```python
from build123d import *

# Parameters (mm, degrees)
SKETCH_1_R      = 1.5
EXTRUDE_1_DEPTH = 42
SKETCH_2_R      = 1.25
EXTRUDE_2_DEPTH = 0.8
SKETCH_3_R      = 1.5
EXTRUDE_3_DEPTH = 3
SKETCH_4_R      = 2.8
EXTRUDE_4_DEPTH = 1.3
FILLET_1_R      = 1


with BuildPart() as part:
    # 草图1 → 凸台-拉伸1 (new body)
    with BuildSketch(Plane(origin=(0, 0, 0), x_dir=(1, 0, 0), z_dir=(0, 1, 0))):
        with Locations(Location((0, 0, 0), (0, 0, 90))):
            Circle(SKETCH_1_R)
    extrude(amount=EXTRUDE_1_DEPTH)

    # 草图2 → 凸台-拉伸2 (add)
    with BuildSketch(Plane(origin=(0, 42, 0), x_dir=(1, 0, 0), z_dir=(0, 1, 0))):
        with Locations(Location((0, 0, 0), (0, 0, 270))):
            Circle(SKETCH_2_R)
    extrude(amount=EXTRUDE_2_DEPTH)

    # 草图3 → 凸台-拉伸3 (add)
    with BuildSketch(Plane(origin=(0, 42.8, 0), x_dir=(1, 0, 0), z_dir=(0, 1, 0))):
        with Locations(Location((0, 0, 0), (0, 0, 90))):
            Circle(SKETCH_3_R)
    extrude(amount=EXTRUDE_3_DEPTH)

    # 草图4 → 凸台-拉伸4 (add)
    with BuildSketch(Plane.XZ):
        with Locations(Location((0, 0, 0), (0, 0, 270))):
            Circle(SKETCH_4_R)
    extrude(amount=EXTRUDE_4_DEPTH)

    # 圆角1
    fillet_1_edges = [part.edges().sort_by_distance(p)[0] for p in [
        (0, -1.3, 2.8),
    ]]
    fillet(fillet_1_edges, radius=FILLET_1_R)


solid = part.part
```
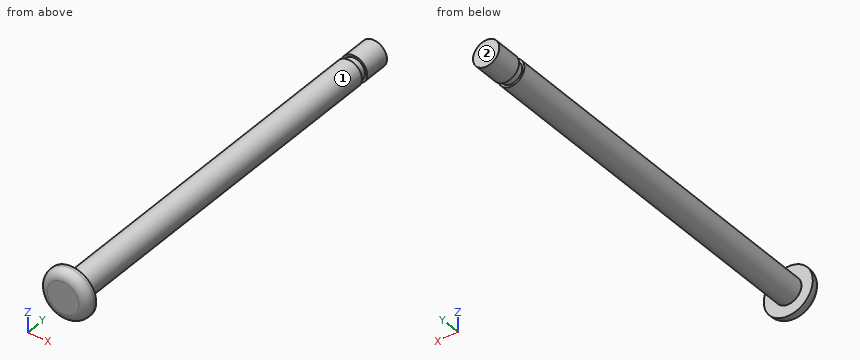
Model file for the job. Use its own axes, mm. Face numbers are marked on the shaded views. A direction names the side the tool comes from. Round coordinates to 2 decimals unless told otherwise and drop trailing zeros. Order: outer loops, then holes, each group sorted by start corner. A loop starts at its lowest first (then second) coordinate and runs counter-clockwise, first axis right, second up. Notation, with made-up numbers: M 72,62 L 77,62 A25 cw 77,92 Z; hole C 23.5,0 d6. An arc over 180 degrees is marked long. Use CSV: the item, a comma, the result in double quotes.
Item 1: Which spindle directions (+Z, -Z, +X, -X, +Y, -Y) get a long thin tool onto all of the face, cutting with end or side? Do the marked faces 1 and 2. Say none if no direction does.
Worked answers:
face 1,"+Y"
face 2,"+Z, -Z, +X, -X, +Y"
Item 2: Saw through at C-C (y = 13.5). List the corners of the cut face in (x, z), plus the area to 3 significant figures.
Worked answers:
outline,"C 0,0 d3"
area,"7.07 mm²"
Item 3: Saw through at B-B (z = 0). List the corners of the cut face in (x, y).
Worked answers:
outline,"M -2.8,-0.3 A1 ccw -1.8,-1.3 L 1.8,-1.3 A1 ccw 2.8,-0.3 L 2.8,0 L 1.5,0 L 1.5,42 L 1.25,42 L 1.25,42.8 L 1.5,42.8 L 1.5,45.8 L -1.5,45.8 L -1.5,42.8 L -1.25,42.8 L -1.25,42 L -1.5,42 L -1.5,0 L -2.8,0 Z"
Item 4: Saw through at A-A (x = 0). List the corners of the cut face in (y, z), plus the area to 3 significant figures.
Worked answers:
outline,"M -1.3,-1.8 A1 ccw -0.3,-2.8 L 0,-2.8 L 0,-1.5 L 42,-1.5 L 42,-1.25 L 42.8,-1.25 L 42.8,-1.5 L 45.8,-1.5 L 45.8,1.5 L 42.8,1.5 L 42.8,1.25 L 42,1.25 L 42,1.5 L 0,1.5 L 0,2.8 L -0.3,2.8 A1 ccw -1.3,1.8 Z"
area,"144 mm²"
Item 5: Pin check, flat tips, straight feed: pin 1 (3 mm diameter, centred on x = 1.5, y = 18, fed in from +Z); pin 2 (3 mm diameter, centred on y = 31.5, z = -1.5, fed in from -X); pin 3 (3 mm diameter, centred on y = 22.5, z = 0.5, fed in from +X). Stop position of each tip, or through.
Worked answers:
pin 1,"z = 1.5"
pin 2,"x = -1.5"
pin 3,"x = 1.5"
Item 6: Probe probe 1 along X at (y, z) = (14, 0.1); probe 2 along Y at (x, z) = (-0.65, 1.7); probe 3 along Z at (x, y) = (0.55, 30.5). List the from-to ranges inside material, lowest first.
Worked answers:
probe 1,"-1.5 to 1.5"
probe 2,"-1.3 to 0"
probe 3,"-1.4 to 1.4"
